Source: CAD feature listing. Evaluate the final solid. Frame: model axes, mm. A direction names the side the tool comes from. Round coordinates to 2 decimals unless told otherwise and drop trailing zeros. Write each loop counter-clockwise with the first axis right and the second up, starting at its lowest first coordinate (ties: lowest second). Pieces come first, ordered by that corner, then holes.
```python
from build123d import *

# Parameters (mm, degrees)
SKETCH1_R                = 17
BOSS_EXTRUDE1_DEPTH      = 10
CUT_EXTRUDE2_REACH       = 28.038
BOSS_EXTRUDE2_DEPTH      = 11
BOSS_EXTRUDE2_DEPTH_BACK = 1
SKETCH1_6_R              = 17
SKETCH1_6_R_2            = 15
CUT_EXTRUDE3_REACH       = 28.439
SKETCH1_7_R              = 2.5


with BuildPart() as part:
    # Sketch1 → Boss-Extrude1 (new body)
    with BuildSketch(Plane.XY):
        Circle(SKETCH1_R)
    extrude(amount=BOSS_EXTRUDE1_DEPTH)

    # Sketch1_5 → Cut-Extrude2 (cut, up to next)
    with BuildSketch(Plane.XY, mode=Mode.PRIVATE) as cut_extrude2_sk1:
        with BuildLine():
            Line((7.5, 12.990381057), (2.5, 4.330127019))
            ThreePointArc((2.5, 4.330127019), (4.330127019, 2.5), (5, 0))
            Line((5, 0), (15, 0))
            ThreePointArc((15, 0), (12.990381057, 7.5), (7.5, 12.990381057))
        make_face()
    cut_extrude2_tool1 = extrude(cut_extrude2_sk1.sketch, amount=CUT_EXTRUDE2_REACH, mode=Mode.PRIVATE) & part.part
    # Sketch1_5 → Cut-Extrude2 (cut, up to next)
    with BuildSketch(Plane.XY, mode=Mode.PRIVATE) as cut_extrude2_sk2:
        with BuildLine():
            Line((7.5, -12.990381057), (2.5, -4.330127019))
            ThreePointArc((2.5, -4.330127019), (0, -5), (-2.5, -4.330127019))
            Line((-2.5, -4.330127019), (-7.5, -12.990381057))
            ThreePointArc((-7.5, -12.990381057), (0, -15), (7.5, -12.990381057))
        make_face()
    cut_extrude2_tool2 = extrude(cut_extrude2_sk2.sketch, amount=CUT_EXTRUDE2_REACH, mode=Mode.PRIVATE) & part.part
    # Sketch1_5 → Cut-Extrude2 (cut, up to next)
    with BuildSketch(Plane.XY, mode=Mode.PRIVATE) as cut_extrude2_sk3:
        with BuildLine():
            ThreePointArc((-5, 0), (-4.330127019, 2.5), (-2.5, 4.330127019))
            Line((-2.5, 4.330127019), (-7.5, 12.990381057))
            ThreePointArc((-7.5, 12.990381057), (-12.990381057, 7.5), (-15, 0))
            Line((-15, 0), (-5, 0))
        make_face()
    cut_extrude2_tool3 = extrude(cut_extrude2_sk3.sketch, amount=CUT_EXTRUDE2_REACH, mode=Mode.PRIVATE) & part.part
    add(cut_extrude2_tool1.solids().sort_by_distance((8.959095, 5.172536, 0))[0], mode=Mode.SUBTRACT)
    add(cut_extrude2_tool2.solids().sort_by_distance((0, -10.345071, 0))[0], mode=Mode.SUBTRACT)
    add(cut_extrude2_tool3.solids().sort_by_distance((-8.959095, 5.172536, 0))[0], mode=Mode.SUBTRACT)

    # Sketch1_6 → Boss-Extrude2 (add, two sides: drawn at the far end of the back side and taken through both)
    with BuildSketch(Plane.XY.offset(-BOSS_EXTRUDE2_DEPTH_BACK)):
        Circle(SKETCH1_6_R)
        Circle(SKETCH1_6_R_2, mode=Mode.SUBTRACT)
    extrude(amount=BOSS_EXTRUDE2_DEPTH + BOSS_EXTRUDE2_DEPTH_BACK)

    # Sketch1_7 → Cut-Extrude3 (cut, up to next)
    with BuildSketch(Plane.XY, mode=Mode.PRIVATE) as cut_extrude3_sk1:
        Circle(SKETCH1_7_R)
    cut_extrude3_tool1 = extrude(cut_extrude3_sk1.sketch, amount=CUT_EXTRUDE3_REACH, mode=Mode.PRIVATE) & part.part
    add(cut_extrude3_tool1.solids().sort_by_distance((0, 0, 0))[0], mode=Mode.SUBTRACT)


solid = part.part
```
Q1. Mould query, pull axis X, two halves, no side actions, for faces 4 (the face through (5.035, -8.721, 4.93)), 5 (the face through (9.139, 14.334, 4.916)), 6 (the face through (6, -14, 11)). Classes: pulls with the +X half, pulls with the -X half, needs draft (parallel to the pull), parting line crosses it, or undercut.
Q2. Section query A-A, the plane x = 0. Output: boundary loops of the cut face in (y, z), and give its area (3 significant figures).
Q3. Section query B-B, the plane y = -6.5. Output: boundary loops of the cut face in (x, z), and give its area (3 significant figures).
Q4. Set-up query: faces 1 (the face through (10, 0, 5)), 2 (the face through (3, 1, 0)), 3 (the face through (3, 1, 10)). Return all of +Z, -Z, +X, -X, +Y, -Y with unobstructed straight access to the full face (end or side cutting, diameter ignored); none if empty.
Q5. Section query D-D, the plane x = -8.5. Output: boundary loops of the cut face in (y, z).
Q6. Section query C-C, the plane z = 1.5. Output: boundary loops of the cut face in (x, y), and give its area (3 significant figures).
Q7. Line query: line 1 (Y direction, x = 0, z = 3.75); line 2 (Y direction, x = 6.5, z = 2.5); line 3 (X direction, y = 3, z = 3.5). Output: solid intervals per line, ascending.
Q8. Pin query (flat end, axial travel): P1, Ø1, axis at x = 9, y = -2, coming from the +Z side; P2, Ø4, axis at y = -4, z = 1.5, coming from the -X side; P3, Ø4, axis at x = -13, z = 5.5, coming from the +Y side; P4, Ø6, axis at x = -1, z = 2, coming from the -Y side. Return the tip coordinate at first contact, or that it passes through.
Filled in:
1. face 4: undercut
1. face 5: parting line crosses it
1. face 6: needs draft
2. outline: (-17, -1) - (-15, -1) - (-15, 11) - (-17, 11) - close; (-5, 0) - (-2.5, 0) - (-2.5, 10) - (-5, 10) - close; (2.5, 0) - (15, 0) - (15, -1) - (17, -1) - (17, 11) - (15, 11) - (15, 10) - (2.5, 10) - close
2. area: 198 mm2
3. outline: (-15.71, -1) - (-13.52, -1) - (-13.52, 0) - (-3.75, 0) - (-3.75, 10) - (-13.52, 10) - (-13.52, 11) - (-15.71, 11) - close; (3.75, 0) - (13.52, 0) - (13.52, -1) - (15.71, -1) - (15.71, 11) - (13.52, 11) - (13.52, 10) - (3.75, 10) - close
3. area: 248 mm2
4. face 1: +Z, -Z
4. face 2: -Z
4. face 3: +Z
5. outline: (-14.72, -1) - (-12.36, -1) - (-12.36, 0) - (0, 0) - (0, 10) - (-12.36, 10) - (-12.36, 11) - (-14.72, 11) - close; (12.36, -1) - (14.72, -1) - (14.72, 11) - (12.36, 11) - close
6. outline: circle Ø34 at (0, 0); hole (-15, 0) - (-5, 0) arc R5 cw to (-2.5, 4.33) - (-7.5, 12.99) arc R15 ccw to start; hole (-7.5, -12.99) arc R15 ccw to (7.5, -12.99) - (2.5, -4.33) arc R5 cw to (-2.5, -4.33) - close; hole circle Ø5 at (0, 0); hole (2.5, 4.33) arc R5 cw to (5, 0) - (15, 0) arc R15 ccw to (7.5, 12.99) - close
6. area: 574 mm2
7. line 1: y = -17 to -15, -5 to -2.5, 2.5 to 17
7. line 2: y = -15.71 to -13.52, -11.26 to 0, 11.26 to 15.71
7. line 3: x = -16.73 to -14.7, -4 to 4, 14.7 to 16.73
8. P1: stops at z = 10
8. P2: stops at x = -16.88
8. P3: stops at y = 12.96
8. P4: stops at y = -17
